```python
from build123d import *

# Parameters (mm, degrees)
SKETCH1_R           = 31
SKETCH1_R_2         = 12.5
BOSS_EXTRUDE1_DEPTH = 8.5
SKETCH3_R           = 26.35
SKETCH3_R_2         = 18.3
CUT_EXTRUDE1_DEPTH  = 2
BOSS_EXTRUDE2_START = -1.7
SKETCH4_R           = 33.85
SKETCH4_R_2         = 31
BOSS_EXTRUDE2_DEPTH = 1.7


with BuildPart() as part:
    # Sketch1 → Boss-Extrude1 (new, symmetric)
    with BuildSketch(Plane.XY):
        Circle(SKETCH1_R)
        Circle(SKETCH1_R_2, mode=Mode.SUBTRACT)
    extrude(amount=BOSS_EXTRUDE1_DEPTH, both=True)

    # Sketch3 → Cut-Extrude1 (cut)
    with BuildSketch(Plane.XY.offset(8.5)):
        Circle(SKETCH3_R)
        Circle(SKETCH3_R_2, mode=Mode.SUBTRACT)
    cut_extrude1 = extrude(amount=-CUT_EXTRUDE1_DEPTH, mode=Mode.SUBTRACT)

    # Mirror1: Cut-Extrude1 across plane
    add(cut_extrude1.mirror(Plane.XY), mode=Mode.SUBTRACT)

    # Sketch4 → Boss-Extrude2 (add)
    with BuildSketch(Plane(origin=(0, 0, -5), x_dir=(-1, 0, 0), z_dir=(0, 0, -1)).offset(BOSS_EXTRUDE2_START)):
        Circle(SKETCH4_R)
        Circle(SKETCH4_R_2, mode=Mode.SUBTRACT)
    extrude(amount=BOSS_EXTRUDE2_DEPTH)


solid = part.part
```
The model under review builds one solid part; all positions refer to its coordinate system, in mm. A direction names the side the tool comes from. Round coordinates to 2 decimals unless told otherwise and drop trailing zeros. Order: outer loops, then holes, each group sorted by start corner. A loop starts at its lowest first (then second) coordinate and runs counter-clockwise, first axis right, second up.
Item 1: For pin 1 (1 mm diameter, centred on y = 6, z = -4.5, fed in from +X); pin 2 (20.5 mm diameter, centred on x = 5, y = -6, fed in from +Z); pin 3 (8 mm diameter, centred on y = 12, z = -3.5, fed in from +X); pin 4 (6 mm diameter, centred on y = -26.5, z = 5, fed in from -X), all flat-tipped, find the tip position at first contact; note any pin that passes through.
Working result:
pin 1: stops at x = 33.4
pin 2: stops at z = 8.5
pin 3: stops at x = 32.89
pin 4: stops at x = -20.22
Item 2: Machinability: for faces 1 (the flat face through (-14.9, -27.4, -3.3)), 2 (the flat face through (-4.3, -11.9, -8.5)), 3 (the cylindrical face through (-5.712, -25.723, -7.514)), which of the approach directions +Z, -Z, +X, -X, +Y, -Y give a long, thin tool a straight path to every point of the face, cutting with its end or side? Answer none if there is none.
Working result:
face 1: +Z
face 2: -Z, +X, -X, +Y, -Y
face 3: -Z
Item 3: Add section D-D, the plane z = 3.5. State the section outline as (x, y) points.
Working result:
outline: circle Ø62 at (0, 0); hole circle Ø25 at (0, 0)
Item 4: To check wall thickness, follow probe 1 along Y at (x, z) = (0, 7.55); probe 2 along Y at (x, z) = (0, 0); probe 3 along Y at (x, z) = (-6, 7.5). State the ranges of each line that lie inside material, in increasing order.
Working result:
probe 1: y = -31 to -26.35, -18.3 to -12.5, 12.5 to 18.3, 26.35 to 31
probe 2: y = -31 to -12.5, 12.5 to 31
probe 3: y = -30.41 to -25.66, -17.29 to -10.97, 10.97 to 17.29, 25.66 to 30.41
Item 5: Add section C-C, the plane z = -7.5. State the section outline as (x, y) points.
Working result:
outline: circle Ø62 at (0, 0); circle Ø36.6 at (0, 0); hole circle Ø52.7 at (0, 0); hole circle Ø25 at (0, 0)
Item 6: Draft analysis for pull direction X (two halves, no side actions). For faces 4 (the cylindrical face through (-4.036, 30.736, -6.726)), 5 (the flat face through (-4.3, -11.9, 8.5)), 6 (the cylindrical face through (9.84, 15.43, -7.51)), state which applies: released by +X, released by -X, zero draft, split by the parting line, or undercut.
Working result:
face 4: split by the parting line
face 5: zero draft
face 6: undercut
